```python
from build123d import *

# Parameters (mm, degrees)
BOSS_EXTRUDE1_DEPTH                              = 270
CUT_EXTRUDE1_DEPTH                               = 271.477244884
F_0_4_0_4_DIAMETER_HOLE1_D                       = 0.4
CBORE_FOR_M4_HEX_HEAD_MACHINE_SCREW1_D           = 4.5
CBORE_FOR_M4_HEX_HEAD_MACHINE_SCREW1_DEPTH       = 4.1
CBORE_FOR_M4_HEX_HEAD_MACHINE_SCREW1_CBORE_D     = 8.5
CBORE_FOR_M4_HEX_HEAD_MACHINE_SCREW1_CBORE_DEPTH = 3.1
FILLET1_R                                        = 0.2
FILLET2_R                                        = 0.5
FILLET3_R                                        = 1
CUT_EXTRUDE2_REACH                               = 302.339
SKETCH7_R                                        = 2.5


with BuildPart() as part:
    # Sketch1 → Boss-Extrude1 (new body)
    with BuildSketch(Plane(origin=(0, 300, 0), x_dir=(1, 0, 0), z_dir=(0, 1, 0))):
        with BuildLine():
            Line((-13.5, -3), (-13.5, -8.7))
            Line((-13.5, -8.7), (13.5, -8.7))
            Line((13.5, -8.7), (13.5, -3))
            Line((13.5, -3), (7.8, -3))
            ThreePointArc((7.8, -3), (7.05, -2.25), (7.8, -1.5))
            Line((7.8, -1.5), (11, -1.5))
            Line((11, -1.5), (11, 0))
            Line((11, 0), (-11, 0))
            Line((-11, 0), (-11, -1.5))
            Line((-11, -1.5), (-7.8, -1.5))
            ThreePointArc((-7.8, -1.5), (-7.05, -2.25), (-7.8, -3))
            Line((-7.8, -3), (-13.5, -3))
        make_face()
    extrude(amount=-BOSS_EXTRUDE1_DEPTH)

    # Sketch2 → Cut-Extrude1 (cut, through all)
    with BuildSketch(Plane.XZ.offset(-30)):
        Polygon((8.75, 8.7), (-8.75, 8.7), (-8.75, 7.6), (-12, 7.6), (-12, 4.1), (12, 4.1), (12, 7.6), (8.75, 7.6), align=None)
    extrude(amount=-CUT_EXTRUDE1_DEPTH, mode=Mode.SUBTRACT)

    # Ø0.4 (0.4) Diameter Hole1 (through all)
    with Locations(Plane(origin=(0, 300, 0), x_dir=(1, 0, 0), z_dir=(0, 1, 0))):
        with Locations((-7.75, -4.1), (7.75, -4.1)):
            Hole(F_0_4_0_4_DIAMETER_HOLE1_D / 2)

    # CBORE for M4 Hex Head Machine Screw1
    with Locations(Plane.XY.offset(4.1)):
        with Locations((0, 260), (0, 200), (0, 140), (0, 80), (0, 20)):
            CounterBoreHole(CBORE_FOR_M4_HEX_HEAD_MACHINE_SCREW1_D / 2, CBORE_FOR_M4_HEX_HEAD_MACHINE_SCREW1_CBORE_D / 2, CBORE_FOR_M4_HEX_HEAD_MACHINE_SCREW1_CBORE_DEPTH, depth=CBORE_FOR_M4_HEX_HEAD_MACHINE_SCREW1_DEPTH)

    # Fillet1
    fillet1_edges = [part.edges().sort_by_distance(p)[0] for p in [
        (-11, 165, 1.5),
        (11, 165, 1.5),
    ]]
    fillet(fillet1_edges, radius=FILLET1_R)

    # Fillet2
    fillet2_edges = [part.edges().sort_by_distance(p)[0] for p in [
        (12, 165, 7.6),
        (12, 165, 4.1),
        (-12, 165, 4.1),
        (-12, 165, 7.6),
    ]]
    fillet(fillet2_edges, radius=FILLET2_R)

    # Fillet3
    fillet3_edges = [part.edges().sort_by_distance(p)[0] for p in [
        (13.5, 165, 3),
        (13.5, 165, 8.7),
        (-13.5, 165, 8.7),
        (-13.5, 165, 3),
    ]]
    fillet(fillet3_edges, radius=FILLET3_R)

    # Sketch7 → Cut-Extrude2 (cut, up to next)
    with BuildSketch(Plane.XY.offset(4.1), mode=Mode.PRIVATE) as cut_extrude2_sk1:
        with Locations((0, 285)):
            Circle(SKETCH7_R)
    cut_extrude2_tool1 = extrude(cut_extrude2_sk1.sketch, amount=-CUT_EXTRUDE2_REACH, mode=Mode.PRIVATE) & part.part
    # Sketch7 → Cut-Extrude2 (cut, up to next)
    with BuildSketch(Plane.XY.offset(4.1), mode=Mode.PRIVATE) as cut_extrude2_sk2:
        with Locations((0, 45)):
            Circle(SKETCH7_R)
    cut_extrude2_tool2 = extrude(cut_extrude2_sk2.sketch, amount=-CUT_EXTRUDE2_REACH, mode=Mode.PRIVATE) & part.part
    # Sketch7 → Cut-Extrude2 (cut, up to next)
    with BuildSketch(Plane.XY.offset(4.1), mode=Mode.PRIVATE) as cut_extrude2_sk3:
        with Locations((0, 35)):
            Circle(SKETCH7_R)
    cut_extrude2_tool3 = extrude(cut_extrude2_sk3.sketch, amount=-CUT_EXTRUDE2_REACH, mode=Mode.PRIVATE) & part.part
    # Sketch7 → Cut-Extrude2 (cut, up to next)
    with BuildSketch(Plane.XY.offset(4.1), mode=Mode.PRIVATE) as cut_extrude2_sk4:
        with Locations((0, 295)):
            Circle(SKETCH7_R)
    cut_extrude2_tool4 = extrude(cut_extrude2_sk4.sketch, amount=-CUT_EXTRUDE2_REACH, mode=Mode.PRIVATE) & part.part
    add(cut_extrude2_tool1.solids().sort_by_distance((0, 285, 4.1))[0], mode=Mode.SUBTRACT)
    add(cut_extrude2_tool2.solids().sort_by_distance((0, 45, 4.1))[0], mode=Mode.SUBTRACT)
    add(cut_extrude2_tool3.solids().sort_by_distance((0, 35, 4.1))[0], mode=Mode.SUBTRACT)
    add(cut_extrude2_tool4.solids().sort_by_distance((0, 295, 4.1))[0], mode=Mode.SUBTRACT)


solid = part.part
```
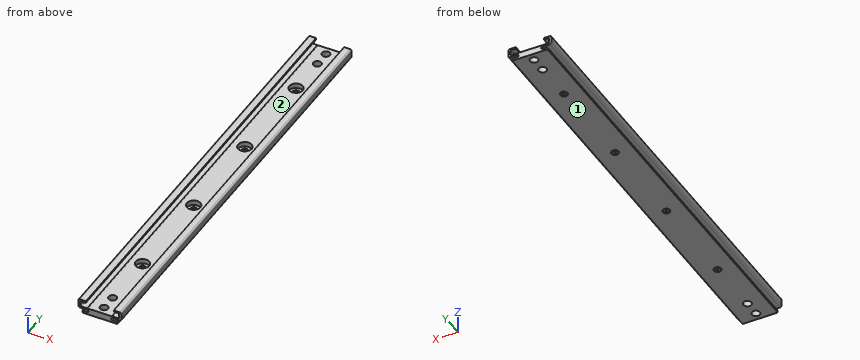
Geometry: final body of the model. Coordinates: model frame, mm. Face numbers are marked on the shaded views. A direction names the side the tool comes from. Round coordinates to 2 decimals unless told otherwise and drop trailing zeros. Use CSV: the item, a comma, the result in double quotes. Start each with the question number.
Q1. Access query for the marked faces 1 and 2. Directions: +Z, -Z, +X, -X, +Y, -Y. A direction counts if a zero-diameter tool reaches every point of the face in a straight line with its end or side. Return the directions, or none.
Q2. First-contact query: pin 1 (4.5 mm diameter, centred on x = -1.5, y = 201.5, fed in from +Z); pin 2 (1.4 mm diameter, centred on y = 183.5, z = 0.5, fed in from -X); pin 3 (5 mm diameter, centred on y = 204, z = 1, fed in from -X); pin 4 (4 mm diameter, centred on x = 0, y = 200, fed in from -Z). Flat tips, straight axial feed; report the tip coordinate or a pass-through.
Q3. Material intervals for line 1 along Z through (x, y) = (-10.25, 190); line 2 along X through (y, z) = (260, 2.3); line 3 along X through (y, z) = (125, 4.5), sorted ascending. Write a range as from..to.
Result set:
1,face 1,"-Z, +X, -X, +Y, -Y"
1,face 2,"+Z, +Y, -Y"
2,pin 1,"stops at z = 4.1"
2,pin 2,"stops at x = -11"
2,pin 3,"stops at x = -13.37"
2,pin 4,"passes through"
3,line 1,"z = 0..1.5, 3..4.1, 7.6..8.7"
3,line 2,"x = -7.05..-4.25, 4.25..7.05"
3,line 3,"x = -13.5..-11.99, 11.99..13.5"
